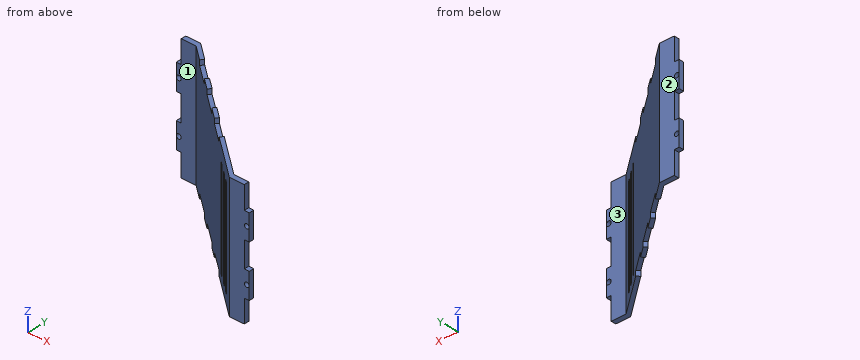
```python
from build123d import *

# Parameters (mm, degrees)
F0_W     = 12.7
F0_H     = 3.175
F1_DEPTH = 39.37
F2_W     = 3.175
F2_H     = 14.605
F2_H_2   = 16.51
F2_R     = 1.5
F3_DEPTH = 25.4
F4_W     = 3.175
F4_H     = 14.605
F4_R     = 1.5
F5_DEPTH = 25.4
F6_W     = 3.175
F6_H     = 63.5
F6_W_2   = 16.51
F6_H_2   = 3.175
F7_DEPTH = 25.4


with BuildPart() as f1:
    # F0 (on Top) → F1 (new body, symmetric)
    with BuildSketch(Plane.XY):
        with Locations((-50.2026024774, 36.647943407)):
            Rectangle(F0_W, F0_H)
        Polygon((-43.8526024774, 38.235443407), (-43.8526024774, 35.060443407), (43.8526024774, -38.235443407), (43.8526024774, -35.060443407), align=None)
        with Locations((50.2026024774, -36.647943407)):
            Rectangle(F0_W, F0_H)
    extrude(amount=F1_DEPTH, both=True)

    # F2 (on face) → F3 (cut)
    with BuildSketch(Plane(origin=(0, 38.235443407, 0), x_dir=(-1, 0, 0), z_dir=(0, 1, 0))):
        with Locations((54.9651024774, 32.0675)):
            Rectangle(F2_W, F2_H)
        with Locations((54.9651024774, 0)):
            Rectangle(F2_W, F2_H_2)
        with Locations((54.9651024774, -32.0675)):
            Rectangle(F2_W, F2_H)
        with Locations((54.9651024774, 16.51)):
            Circle(F2_R)
        with Locations((54.9651024774, -16.51)):
            Circle(F2_R)
    extrude(amount=-F3_DEPTH, mode=Mode.SUBTRACT)

    # F4 (on face) → F5 (cut)
    with BuildSketch(Plane(origin=(0, -35.060443407, 0), x_dir=(-1, 0, 0), z_dir=(0, 1, 0))):
        with Locations((-54.9651024774, 32.0675)):
            Rectangle(F4_W, F4_H)
        with Locations((-54.9651024774, -32.0675)):
            Rectangle(F4_W, F4_H)
        Polygon((-56.5526024774, 8.255), (-56.5526024774, 0), (-56.5526024774, -8.255), (-53.3776024774, -8.255), (-53.3776024774, 8.255), align=None)
        with Locations((-54.9651024774, 16.51)):
            Circle(F4_R)
        with Locations((-54.9651024774, -16.51)):
            Circle(F4_R)
    extrude(amount=-F5_DEPTH, mode=Mode.SUBTRACT)

    # F6 (on face) → F7 (cut)
    with BuildSketch(Plane(origin=(0.7811352648, 0.9346994965, 0), x_dir=(-0.7673246278, 0.6412588523, 0), z_dir=(0.6412588523, 0.7673246278, 0))):
        with Locations((-31.684501572, -1.7767186165)):
            Rectangle(F6_W, F6_H)
        with Locations((-39.304501572, -1.7767186165)):
            Rectangle(F6_W, F6_H)
        with Locations((-46.924501572, -1.7767186165)):
            Rectangle(F6_W, F6_H)
        with Locations((35.942998428, 37.7825)):
            Rectangle(F6_W_2, F6_H_2)
        with Locations((10.542998428, 37.7825)):
            Rectangle(F6_W_2, F6_H_2)
        with Locations((-14.857001572, 37.7825)):
            Rectangle(F6_W_2, F6_H_2)
        with Locations((35.942998428, -37.7825)):
            Rectangle(F6_W_2, F6_H_2)
        with Locations((10.542998428, -37.7825)):
            Rectangle(F6_W_2, F6_H_2)
        with Locations((-14.857001572, -37.7825)):
            Rectangle(F6_W_2, F6_H_2)
    extrude(amount=-F7_DEPTH, mode=Mode.SUBTRACT)


solid = f1.part
```
The listing builds one solid part. Answer for the finished solid, in the listing's coordinates (mm). Face numbers are marked on the shaded views. A direction names the side the tool comes from. Round coordinates to 2 decimals unless told otherwise and drop trailing zeros. Loops run counter-clockwise (first coordinate to the right, second up) from the corner with the lowest first, then second, coordinate; pieces in that order, holes last. Notation, with made-up numbers: (4.5, -1) - (27.5, -1) arc R26 ccw to (27.5, 15) - close; hole circle Ø7 at (41, -22.5). An arc over 180 degrees is marked (long way). Return JSON: item names as keys, results as strings. Group by question number.
1. The part is cut by section D-D on y = 20. Determine the outline of the cut face in (x, z) (3 decimals), then the cut area to 3 significant figures.
2. Consider probe 1 along Z at (x, y) = (-9.5, 9) (3 decimals); probe 2 along Y at (x, z) = (-44, -9.5); probe 3 along X at (y, z) = (36, -16). Determine where each line is inside the solid, lowest interval first.
3. Each of these flat-tipped pins is pushed along its axis until it touches: P1, Ø3.5, axis at x = 55.5, y = -36.5, coming from the +Z side (3 decimals); P2, Ø1.5, axis at y = 17, z = 16.5, coming from the +X side (3 decimals); P3, Ø14, axis at x = 51.5, z = 6.5, coming from the +Y side; P4, Ø6, axis at x = 21, y = -11.5, coming from the +Z side. Where does it stop, or does it pass through?
4. The part is cut by section C-C on x = -38.5. Determine the outline of the cut face in (y, z), then the cut area to 3 significant figures.
5. The part is cut by section A-A on z = -16.51. Determine the outline of the cut face in (x, y), then the cut area to 3 significant figures.
6. Which of the six approach directions +Z, -Z, +X, -X, +Y, -Y give full straight-line access (tool end or side, diameter ignored) to the marked faces 1, 2 and 3?
7. The part is cut by section B-B on z = 1. Determine the outline of the cut face in (x, y).
Resolved:
{
 "1": {"outline": "(-25.831, -36.195) - (-22.032, -36.195) - (-22.032, 36.195) - (-25.831, 36.195) - close", "area": "275 mm²"},
 "2": {"probe 1": "z = -36.195 to 36.195", "probe 2": "y = 35.06 to 38.24", "probe 3": "x = -56.55 to -56.38, -53.55 to -41.18"},
 "3": {"P1": "stops at z = 24.765", "P2": "stops at x = -17.545", "P3": "stops at y = -35.06", "P4": "passes through"},
 "4": {"outline": "(30.59, -39.37) - (33.76, -39.37) - (33.76, 39.37) - (30.59, 39.37) - close", "area": "250 mm²"},
 "5": {"outline": "(-56.55, 35.06) - (-56.47, 35.06) - (-56.47, 38.24) - (-56.55, 38.24) - close; (-53.47, 35.06) - (-43.85, 35.06) - (22.31, -20.23) - (23.88, -18.37) - (-43.85, 38.24) - (-53.47, 38.24) - close; (24.75, -22.27) - (28.16, -25.12) - (29.72, -23.25) - (26.31, -20.4) - close; (30.6, -27.16) - (34.01, -30.01) - (35.57, -28.14) - (32.16, -25.29) - close; (36.44, -32.04) - (43.85, -38.24) - (53.47, -38.24) - (53.47, -35.06) - (43.85, -35.06) - (38.01, -30.17) - close; (56.47, -38.24) - (56.55, -38.24) - (56.55, -35.06) - (56.47, -35.06) - close", "area": "317 mm²"},
 "6": {"face 1": "+Z, -Z, -X, -Y", "face 2": "+Z, -Z, +X, -X, +Y", "face 3": "+Z, -Z, +X, +Y"},
 "7": {"outline": "(-53.38, 35.06) - (-43.85, 35.06) - (22.31, -20.23) - (23.88, -18.37) - (-43.85, 38.24) - (-53.38, 38.24) - close; (24.75, -22.27) - (28.16, -25.12) - (29.72, -23.25) - (26.31, -20.4) - close; (30.6, -27.16) - (34.01, -30.01) - (35.57, -28.14) - (32.16, -25.29) - close; (36.44, -32.04) - (43.85, -38.24) - (53.38, -38.24) - (53.38, -35.06) - (43.85, -35.06) - (38.01, -30.17) - close"}
}
